Autodesk Inventor part; units mm, degrees
ref_plane "YZ Plane" through (0, 0, 0) normal (1, 0, 0) x (0, 1, 0)
ref_plane "XZ Plane" through (0, 0, 0) normal (0, 1, 0) x (-1, 0, 0)
ref_plane "XY Plane" through (0, 0, 0) normal (0, 0, 1) x (1, 0, 0)
sketch "스케치1" plane through (0, 0, 0) normal (0, 0, 1) x (1, 0, 0)
  line L0 (-19.5, -10) -> (19.5, -10)
  line L1 (20, -9.5) -> (20, 9.5)
  line L2 (19.5, 10) -> (-19.5, 10)
  line L3 (-20, 9.5) -> (-20, -9.5)
  circle A0 centre (-17, 7) radius 2
  line L4 (0, -12.143) -> (0, 11.1651)
  line L5 (28.9925, 0) -> (-24.8769, 0)
  circle A1 centre (-10, 0) radius 2.1
  line L6 (-10, 12.7543) -> (-10, -12.5913)
  line L7 (10, -12.5913) -> (10, 12.7543)
  circle A2 centre (10, 0) radius 2.1
  line L8 (-12.65, -10) -> (-12.65, -8.5)
  line L9 (-12.65, -8.5) -> (-14.15, -8.5)
  line L10 (-14.15, -8.5) -> (-14.15, -4.7403)
  line L11 (-5.85, -4.7397) -> (-5.85, -8.5)
  line L12 (-5.85, -8.5) -> (-7.35, -8.5)
  line L13 (-7.35, -8.5) -> (-7.35, -10)
  arc A3 (-5.85, -4.7397) -> (-14.15, -4.7403) centre (-9.9996, -10) ccw
  line L14 (-10, -3.05) -> (-10.25, -3.3047)
  line L15 (-10, -3.05) -> (-9.7398, -3.305)
  line L16 (12.65, -10) -> (12.65, -8.5)
  line L17 (12.65, -8.5) -> (14.15, -8.5)
  line L18 (14.15, -8.5) -> (14.15, -4.7403)
  line L19 (5.85, -4.7397) -> (5.85, -8.5)
  line L20 (5.85, -8.5) -> (7.35, -8.5)
  line L21 (7.35, -8.5) -> (7.35, -10)
  arc A4 (14.15, -4.7403) -> (5.85, -4.7397) centre (9.9996, -10) ccw
  line L22 (10, -3.05) -> (10.25, -3.3047)
  line L23 (10, -3.05) -> (9.7398, -3.305)
  line L24 (-20, 2.65) -> (-18.5, 2.65)
  line L25 (-18.5, 2.65) -> (-18.5, 4.15)
  line L26 (-18.5, 4.15) -> (-14.7403, 4.15)
  line L27 (-14.7397, -4.15) -> (-18.5, -4.15)
  line L28 (-18.5, -4.15) -> (-18.5, -2.65)
  line L29 (-18.5, -2.65) -> (-20, -2.65)
  line L30 (-13.05, 0) -> (-13.305, -0.2602)
  line L31 (-13.05, 0) -> (-13.3047, 0.25)
  arc A5 (-14.7397, -4.15) -> (-14.7403, 4.15) centre (-20, -0.0004) ccw
  line L32 (-7.35, 10) -> (-7.35, 8.5)
  line L33 (-7.35, 8.5) -> (-5.85, 8.5)
  line L34 (-5.85, 8.5) -> (-5.85, 4.7403)
  line L35 (-14.15, 4.7397) -> (-14.15, 8.5)
  line L36 (-14.15, 8.5) -> (-12.65, 8.5)
  line L37 (-12.65, 8.5) -> (-12.65, 10)
  line L38 (-10, 3.05) -> (-10.2602, 3.305)
  line L39 (-10, 3.05) -> (-9.75, 3.3047)
  arc A6 (-14.15, 4.7397) -> (-5.85, 4.7403) centre (-10.0004, 10) ccw
  line L40 (14.7397, -4.15) -> (18.5, -4.15)
  line L41 (18.5, -4.15) -> (18.5, -2.65)
  line L42 (18.5, -2.65) -> (20, -2.65)
  arc A7 (14.7403, 4.15) -> (14.7397, -4.15) centre (20, -0.0004) ccw
  line L43 (20, 2.65) -> (18.5, 2.65)
  line L44 (18.5, 2.65) -> (18.5, 4.15)
  line L45 (18.5, 4.15) -> (14.7403, 4.15)
  line L46 (13.05, 0) -> (13.305, -0.2602)
  line L47 (13.05, 0) -> (13.3047, 0.25)
  line L48 (14.15, 4.7397) -> (14.15, 8.5)
  line L49 (14.15, 8.5) -> (12.65, 8.5)
  line L50 (12.65, 8.5) -> (12.65, 10)
  arc A8 (5.85, 4.7403) -> (14.15, 4.7397) centre (10.0004, 10) ccw
  line L51 (7.35, 10) -> (7.35, 8.5)
  line L52 (7.35, 8.5) -> (5.85, 8.5)
  line L53 (5.85, 8.5) -> (5.85, 4.7403)
  line L54 (10, 3.05) -> (10.2602, 3.305)
  line L55 (10, 3.05) -> (9.75, 3.3047)
  circle A9 centre (-17, -7) radius 2
  circle A10 centre (17, 7) radius 2
  circle A11 centre (17, -7) radius 2
  line L56 (-3.85, -8.5) -> (3.85, -8.5)
  line L57 (3.85, 8.5) -> (-3.85, 8.5)
  line L58 (-4.35, -8.5) -> (4.35, 8.5) construction
  line L59 (4.35, -8.5) -> (-4.35, 8.5) construction
  arc A12 (-3.85, 8.5) -> (-4.35, 8) centre (-3.85, 8) ccw
  arc A13 (4.35, 8) -> (3.85, 8.5) centre (3.85, 8) ccw
  arc A14 (3.85, -8.5) -> (4.35, -8) centre (3.85, -8) ccw
  arc A15 (-4.35, -8) -> (-3.85, -8.5) centre (-3.85, -8) ccw
  line L60 (-4.35, 8) -> (-4.35, 4.1325)
  line L61 (-4.35, -4.3275) -> (-4.35, -8)
  line L62 (4.35, -8) -> (4.35, -4.3275)
  line L63 (4.35, 4.3275) -> (4.35, 8)
  arc A16 (4.4769, -3.9946) -> (4.4769, 3.9946) centre (0, 0) ccw
  arc A17 (-4.35, 4.1325) -> (-4.4769, -3.9946) centre (0, 0) ccw
  arc A18 (-4.35, -4.3275) -> (-4.4769, -3.9946) centre (-4.85, -4.3275) ccw
  arc A19 (4.35, 4.3275) -> (4.4769, 3.9946) centre (4.85, 4.3275) ccw
  arc A20 (4.4769, -3.9946) -> (4.35, -4.3275) centre (4.85, -4.3275) ccw
  arc A21 (-19.5, 10) -> (-20, 9.5) centre (-19.5, 9.5) ccw
  arc A22 (-20, -9.5) -> (-19.5, -10) centre (-19.5, -9.5) ccw
  arc A23 (19.5, -10) -> (20, -9.5) centre (19.5, -9.5) ccw
  arc A24 (20, 9.5) -> (19.5, 10) centre (19.5, 9.5) ccw
  point P0 (20, 10)
  point P1 (20, -10)
  point P2 (-20, 10)
  point P3 (-14.15, -6.6202)
  point P4 (-12.65, -9.25)
  point P5 (-10.0001, -3.3)
  point P6 (14.15, -6.6202)
  point P7 (12.65, -9.25)
  point P8 (10.0001, -3.3)
  point P9 (-19.25, 2.65)
  point P10 (-16.6202, 4.15)
  point P11 (-13.3, 0.0001)
  point P12 (-7.35, 9.25)
  point P13 (-5.85, 6.6202)
  point P14 (-9.9999, 3.3)
  point P15 (13.3, 0.0001)
  point P16 (19.25, 2.65)
  point P17 (16.6202, 4.15)
  point P18 (22.5913, 0)
  point P19 (9.9999, 3.3)
  point P20 (7.35, 9.25)
  point P21 (5.85, 6.6202)
  point P22 (10, 12.5913)
  point P23 (-5.85, -6.6199)
  point P24 (-4.35, -4.1325)
  point P25 (4.35, -4.1325)
  point P26 (4.35, 4.1325)
  point P27 (4.35, 6.1638)
  point P28 (-4.35, 6.0662)
  dimension "d0" = 40
  dimension "d1" = 20
  dimension "d2" = 4
  dimension "d3" = 34
  dimension "d4" = 14
  dimension "d5" = 4.2
  dimension "d6" = 20
  dimension "d8" = 4.2
  dimension "d9" = 20
  dimension "d12" = 1.5
  dimension "d13" = 6.7
  dimension "d14" = 8.3
  dimension "d15" = 5.3
  dimension "d16" = 5.3
  dimension "d17" = 8.3
  dimension "d18" = 6.7
  dimension "d19" = 0.5
  dimension "d20" = 0.25
  dimension "d23" = 180
  dimension "d27" = 180
  dimension "d29" = 1.5
  dimension "d31" = 1.5
  dimension "d32" = 0.5
  dimension "d33" = 0.5
  dimension "d34" = 0.5
  dimension "d35" = 8.7
extrude "돌출1" add sketch "스케치1" along normal blind 1 contours A22 L3 L29 L28 L27 A5 L30 L5 A1 L6 L14 A3 L10 L9 L8 L0 | L13 L12 L11 A3 L15 L6 A1 L5 A17 A18 L61 A15 L56 L4 L0 | L4 L56 A14 L62 A20 A16 L5 A2 L7 L23 A4 L19 L20 L21 L0 | L3 A21 L2 L37 L36 L35 A6 L38 L6 A1 L5 L31 A5 L26 L25 L24 | A1 L6 L39 A6 L34 L33 L32 L2 L4 L57 A12 L60 A17 L5 | L16 L17 L18 A4 L22 L7 A2 L5 L46 A7 L40 L41 L42 L1 A23 L0 | L4 L2 L51 L52 L53 A8 L55 L7 A2 L5 A16 A19 L63 A13 L57 | L7 L54 A8 L48 L49 L50 L2 A24 L1 L43 L44 L45 A7 L47 L5 A2
equation "\"d8\" = d5"
properties part number "20x40 profile"
Design review of the part built by this model. Coordinates are the model's own, in mm. A direction names the side the tool comes from. Coordinates: 2 decimals unless noted, no trailing zeros. Loops run counter-clockwise (first coordinate to the right, second up) from the corner with the lowest first, then second, coordinate; pieces in that order, holes last. Notation, with made-up numbers: M 79,-39 L 117,-39 A25 cw 117,-17 Z; hole C 41.5,89.5 d3. An arc over 180 degrees is marked long. Use one line per item in the form item = value.
(1) Consider section B-B (y = -7). Write out the cut boundary in (x, z), and give its area (3 significant figures).
Return value:
outline = M -20,0 L -19,0 L -19,1 L -20,1 Z; M -15,0 L -14.15,0 L -14.15,1 L -15,1 Z; M -5.85,0 L -4.35,0 L -4.35,1 L -5.85,1 Z; M 4.35,0 L 5.85,0 L 5.85,1 L 4.35,1 Z; M 14.15,0 L 15,0 L 15,1 L 14.15,1 Z; M 19,0 L 20,0 L 20,1 L 19,1 Z
area = 6.70 mm2
(2) Consider section D-D (y = 6.25). Write out the cut boundary in (x, z), and give its area (3 significant figures).
Return value:
outline = M -20,0 L -18.85,0 L -18.85,1 L -20,1 Z; M -15.15,0 L -14.15,0 L -14.15,1 L -15.15,1 Z; M -5.85,0 L -4.35,0 L -4.35,1 L -5.85,1 Z; M 4.35,0 L 5.85,0 L 5.85,1 L 4.35,1 Z; M 14.15,0 L 15.15,0 L 15.15,1 L 14.15,1 Z; M 18.85,0 L 20,0 L 20,1 L 18.85,1 Z
area = 7.28 mm2
(3) For faces 5 (the face through (-19.3, 2.65, 0.5)), 6 (the face through (19.3, 2.65, 0.5)), 7 (the face through (-13.72, 2.34, 0.49)), 8 (the face through (-12.65, 9.2, 0.5)), list the 3-axis set-ups (+Z, -Z, +X, -X, +Y, -Y) from which the entire face can be reached by the end or side of a thin tool; tool diameter is ignored.
Return value:
face_5 = +Z, -Z, -X
face_6 = +Z, -Z, +X
face_7 = +Z, -Z
face_8 = +Z, -Z, +Y
(4) Consider section A-A (x = -17). Write out the cut boundary in (y, z).
Return value:
outline = M -10,0 L -9,0 L -9,1 L -10,1 Z; M -5,0 L -4.15,0 L -4.15,1 L -5,1 Z; M 4.15,0 L 5,0 L 5,1 L 4.15,1 Z; M 9,0 L 10,0 L 10,1 L 9,1 Z
(5) Draft analysis for pull direction Y (two halves, no side actions). For faces 1 (the face through (7.35, -9.2, 0.5)), 2 (the face through (0.1, 10, 0.5)), 3 (the face through (-7.709, -3.704, 0.493)), 4 (the face through (7.653, -3.724, 0.493)), state which applies: pulls with the +Y half, pulls with the -Y half, needs draft (parallel to the pull), parting line crosses it, or undercut.
Return value:
face_1 = needs draft
face_2 = pulls with the +Y half
face_3 = undercut
face_4 = undercut
(6) Consider section C-C (x = 11). Write out the cut boundary in (y, z), and give its area (3 significant figures).
Return value:
outline = M -3.38,0 L -1.85,0 L -1.85,1 L -3.38,1 Z; M 1.85,0 L 3.37,0 L 3.37,1 L 1.85,1 Z
area = 3.06 mm2
(7) For line 1 along Y through (x, z) = (-17, 0.5); line 2 along X through (y, z) = (1.5, 0.8); line 3 along Y through (x, z) = (0.5, 0.4), list the stretches that pass through material, from the lowest coordinate up. Write a range as from..to.
Return value:
line_1 = -10..-9, -5..-4.15, 4.15..5, 9..10
line_2 = -13.47..-11.47, -8.53..-5.81, 5.81..8.53, 11.47..13.47
line_3 = -10..-8.5, 8.5..10
